Can you work these out from the model? Positions are in its coordinate system, mm. Face numbers are marked on the shaded views. A direction names the side the tool comes from. Give positions to 0.01 mm unless a question says otherwise; leave off trailing zeros. Order: outer loops, then holes, each group sorted by start corner. A loop starts at its lowest first (then second) coordinate and runs counter-clockwise, first axis right, second up. Notation, with made-up numbers: M 47,-22 L 52,-22 A21 cw 52,17 Z; hole C 25,-22.75 d10. An arc over 180 degrees is marked long. One line per question, with ' | ' between items. Start each with the question number.
1) For the marked faces 1, 2 and 3, which set-ups out of +Z, -Z, +X, -X, +Y, -Y let a thin tool reach every point of the face, with its end or its side?
2) I'm going to push flat-ended pins straight in: pin 1 Ø4.5 at (x, y) = (21, 4) entering from +Z; pin 2 Ø2.5 at (x, z) = (33.5, -22.5) entering from +Y; pin 3 Ø1.2 at (x, y) = (22, 4.5) entering from -Z; pin 4 Ø0.7 at (x, y) = (25.5, -1) entering from +Z. Where does each tip first touch, or does it pass through?
3) If we section it at A-A, the plane z = -3.5: Please give me the cut outline in (x, y).
4) Please list where these lines run through material, in increasing order: line 1 along X through (y, z) = (0.7, -3.5); line 2 along X through (y, z) = (3.25, -3); line 3 along X through (y, z) = (-0.75, -16). Write a range as [from, to].
5) If we section it at D-D, the plane x = 20: Please give me the cut outline in (y, z), plus the area to 3 significant figures.
6) If we section it at C-C, the plane y = 0.5: Please give me the cut outline in (x, z), plus the area to 3 significant figures.
7) If we section it at B-B, the plane x = 3.5: Please give me the cut outline in (y, z), plus the area to 3 significant figures.
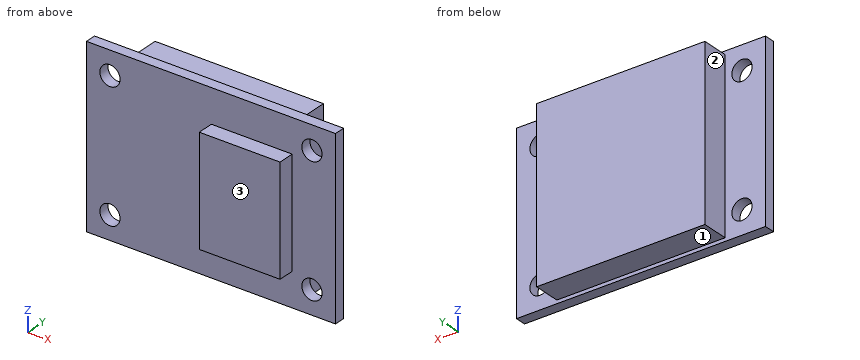
```python
from build123d import *

# Parameters (mm, degrees)
SKETCH1_W           = 37
SKETCH1_H           = 26
SKETCH1_R           = 1.5
BOSS_EXTRUDE1_DEPTH = 1.6
SKETCH2_W           = 25
SKETCH2_H           = 25
BOSS_EXTRUDE2_DEPTH = 4
SKETCH3_W           = 12
SKETCH3_H           = 16
BOSS_EXTRUDE3_DEPTH = 2.4


with BuildPart() as part:
    # Sketch1 → Boss-Extrude1 (new body)
    with BuildSketch(Plane(origin=(0, 0, 0), x_dir=(1, 0, 0), z_dir=(0, 1, 0))):
        with Locations((18.5, 13)):
            Rectangle(SKETCH1_W, SKETCH1_H)
        with Locations(Location((3.5, 22.5, 0), (0, 0, 270))):
            Circle(SKETCH1_R, mode=Mode.SUBTRACT)
        with Locations(Location((33.5, 22.5, 0), (0, 0, 90))):
            Circle(SKETCH1_R, mode=Mode.SUBTRACT)
        with Locations(Location((33.5, 3.5, 0), (0, 0, 270))):
            Circle(SKETCH1_R, mode=Mode.SUBTRACT)
        with Locations(Location((3.5, 3.5, 0), (0, 0, 90))):
            Circle(SKETCH1_R, mode=Mode.SUBTRACT)
    extrude(amount=BOSS_EXTRUDE1_DEPTH)

    # Sketch2 → Boss-Extrude2 (add)
    with BuildSketch(Plane(origin=(0, 1.6, 0), x_dir=(1, 0, 0), z_dir=(0, 1, 0))):
        with Locations((18.5, 13)):
            Rectangle(SKETCH2_W, SKETCH2_H)
    extrude(amount=BOSS_EXTRUDE2_DEPTH)

    # Sketch3 → Boss-Extrude3 (add)
    with BuildSketch(Plane.XZ):
        with Locations((24.565846611, -13)):
            Rectangle(SKETCH3_W, SKETCH3_H)
    extrude(amount=BOSS_EXTRUDE3_DEPTH)


solid = part.part
```
Results found:
1) face 1: -Z, +X, -X, +Y | face 2: +Z, -Z, -X, +Y | face 3: +Z, -Z, +X, -X, -Y
2) pin 1: stops at z = -0.5 | pin 2: passes through | pin 3: stops at z = -25.5 | pin 4: stops at z = -5
3) outline: M 0,0 L 2,0 L 2,1.6 L 0,1.6 Z; M 5,0 L 32,0 L 32,1.6 L 31,1.6 L 31,5.6 L 6,5.6 L 6,1.6 L 5,1.6 Z; M 35,0 L 37,0 L 37,1.6 L 35,1.6 Z
4) line 1: x = [0, 2], [5, 32], [35, 37] | line 2: x = [6, 31] | line 3: x = [18.57, 30.57]
5) outline: M -2.4,-21 L 0,-21 L 0,-26 L 1.6,-26 L 1.6,-25.5 L 5.6,-25.5 L 5.6,-0.5 L 1.6,-0.5 L 1.6,0 L 0,0 L 0,-5 L -2.4,-5 Z | area: 180 mm²
6) outline: M 0,-26 L 37,-26 L 37,0 L 0,0 Z; hole C 3.5,-22.5 d3; hole C 3.5,-3.5 d3; hole C 33.5,-22.5 d3; hole C 33.5,-3.5 d3 | area: 934 mm²
7) outline: M 0,-26 L 1.6,-26 L 1.6,-24 L 0,-24 Z; M 0,-21 L 1.6,-21 L 1.6,-5 L 0,-5 Z; M 0,-2 L 1.6,-2 L 1.6,0 L 0,0 Z | area: 32.0 mm²
